Input: part model. Units: mm. Frame: model coordinates. Give positions to 0.01 mm unless a question says otherwise; leave off trailing zeros. Write each loop counter-clockwise with the first axis right and the second up, starting at its lowest first coordinate (ties: lowest second). Pieces come first, ordered by that corner, then holes. Notation, with made-up numbers: (8, 9) -> (27, 9) arc R29 ccw to (27, 39) -> close; hole circle Ø1 at (61, 45.5). An arc over 180 degrees is marked (long way). Return JSON: item names as keys, results as strings. Group by question number.
Item 1: Section B-B, the plane z = 2. Return loops of the section in (x, y).
Item 2: Section C-C, the plane y = 12.5. Return loops of the section in (x, z) (3 decimals).
Item 3: Line query: line 1 (X direction, y = 34, z = 5.5); line 2 (X direction, y = 21, z = 4.75); line 3 (Y direction, x = 29.5, z = 5.5). Output: solid intervals per line, ascending. Write a range as [from, to].
Item 4: Pin query (flat end, axial travel): P1, Ø3, axis at x = 35, z = 4.5, coming from the -Y side; P2, Ø1, axis at x = 8.5, z = 3, coming from the +Y side. Return the tip coordinate at first contact, or that it passes through.
Item 5: Section A-A, the plane x = 34. Return loops of the section in (y, z) (3 decimals).
Item 6: Section D-D, the plane y = 0. Return loops of the section in (x, z) (3 decimals), then the cut area to 3 significant figures.
from build123d import *

# Parameters (mm, degrees)
F0_R     = 50.8
F1_DEPTH = 6.35
F3_DEPTH = 3.175


with BuildPart() as f1:
    # F0 (on Top) → F1 (new body)
    with BuildSketch(Plane.XY):
        Circle(F0_R)
    extrude(amount=F1_DEPTH)

    # F2 (on face) → F3 (cut)
    with BuildSketch(Plane.XY.offset(6.35)):
        with BuildLine():
            ThreePointArc((15.112324, 8.831488), (3.651467, 2.698075), (-9.320416, 3.53488))
            ThreePointArc((-9.320416, 3.53488), (-32.253054, -21.213472), (-4.365525, -40.204853))
            ThreePointArc((-4.365525, -40.204853), (9.25251, -39.514444), (22.098763, -34.942649))
            ThreePointArc((22.098763, -34.942649), (17.400158, -35.046174), (12.701553, -34.942649))
            ThreePointArc((12.701553, -34.942649), (9.453009, -34.523417), (7.319516, -32.038059))
            ThreePointArc((7.319516, -32.038059), (15.827852, -28.814343), (24.832496, -27.510311))
            ThreePointArc((24.832496, -27.510311), (32.746976, -25.459085), (38.501162, -19.650828))
            ThreePointArc((38.501162, -19.650828), (40.771781, -15.886564), (41.832902, -11.620486))
            ThreePointArc((41.832902, -11.620486), (33.877001, -16.787957), (24.832496, -19.650828))
            ThreePointArc((24.832496, -19.650828), (29.815505, -13.430648), (35.254855, -7.605316))
            ThreePointArc((35.254855, -7.605316), (41.278783, 12.303986), (31.977173, 30.909041))
            ThreePointArc((31.977173, 30.909041), (35.554887, 23.205066), (35.254855, 14.716176))
            ThreePointArc((35.254855, 14.716176), (15.477583, 39.467908), (-16.163122, 41.097168))
            ThreePointArc((-16.163122, 41.097168), (-7.968292, 40.127246), (0, 37.98195))
            ThreePointArc((0, 37.98195), (2.887171, 36.599375), (4.963089, 34.162607))
            ThreePointArc((4.963089, 34.162607), (-1.010732, 31.624663), (-7.500219, 31.505231))
            ThreePointArc((-7.500219, 31.505231), (-1.491468, 29.04792), (4.963089, 29.742295))
            ThreePointArc((4.963089, 29.742295), (7.619099, 31.6133), (10.671567, 32.725722))
            ThreePointArc((10.671567, 32.725722), (14.857029, 32.055581), (17.791109, 28.99644))
            ThreePointArc((17.791109, 28.99644), (19.347167, 23.888888), (18.469164, 18.622248))
            ThreePointArc((18.469164, 18.622248), (15.14181, 21.198982), (12.786984, 24.68691))
            ThreePointArc((12.786984, 24.68691), (17.163098, 13.855457), (27.56623, 8.540798))
            ThreePointArc((27.56623, 8.540798), (26.557747, 5.699635), (26.028505, 2.731615))
            ThreePointArc((26.028505, 2.731615), (24.468311, -0.799827), (21.415329, -3.162999))
            ThreePointArc((21.415329, -3.162999), (20.44222, 2.261754), (21.415329, 7.686506))
            ThreePointArc((21.415329, 7.686506), (19.491688, 5.874092), (18.169021, 3.585906))
            ThreePointArc((18.169021, 3.585906), (16.975731, -0.906667), (16.973011, -5.555016))
            ThreePointArc((16.973011, -5.555016), (16.032075, -11.360599), (12.616124, -16.148232))
            ThreePointArc((12.616124, -16.148232), (6.875784, -18.260537), (2.127092, -14.405247))
            ThreePointArc((2.127092, -14.405247), (3.95514, -10.785374), (7.252841, -8.425204))
            ThreePointArc((7.252841, -8.425204), (13.847913, -1.010771), (15.112324, 8.831488))
        make_face()
        with BuildLine():
            ThreePointArc((-23.696838, 23.682131), (-19.798362, 29.346782), (-13.441595, 31.969357))
            ThreePointArc((-13.441595, 31.969357), (-16.672015, 37.73461), (-23.107406, 36.231447))
            ThreePointArc((-23.107406, 36.231447), (-29.15748, 31.539036), (-32.012127, 24.434594))
            ThreePointArc((-32.012127, 24.434594), (-28.736741, 26.680977), (-25.31456, 28.696684))
            ThreePointArc((-25.31456, 28.696684), (-24.969334, 27.114262), (-24.609111, 25.535187))
            ThreePointArc((-24.609111, 25.535187), (-24.317241, 24.527789), (-23.696838, 23.682131))
        make_face()
        with BuildLine():
            ThreePointArc((-9.197756, 25.535187), (-6.724581, 24.427669), (-5.085402, 22.269826))
            ThreePointArc((-5.085402, 22.269826), (-3.220597, 19.405613), (-0.489241, 17.351128))
            ThreePointArc((-0.489241, 17.351128), (2.029713, 17.241099), (4.510092, 17.693825))
            ThreePointArc((4.510092, 17.693825), (6.713953, 19.342602), (8.158797, 21.685228))
            ThreePointArc((8.158797, 21.685228), (8.296615, 23.240133), (7.715309, 24.688859))
            ThreePointArc((7.715309, 24.688859), (5.068899, 26.392475), (2.212011, 25.071872))
            ThreePointArc((2.212011, 25.071872), (1.166697, 24.006752), (0, 23.076171))
            ThreePointArc((0, 23.076171), (-1.454137, 22.680928), (-2.908273, 23.076171))
            ThreePointArc((-2.908273, 23.076171), (-4.628321, 24.658533), (-6.657773, 25.817741))
            ThreePointArc((-6.657773, 25.817741), (-7.961822, 25.982624), (-9.197756, 25.535187))
        make_face()
    extrude(amount=-F3_DEPTH, mode=Mode.SUBTRACT)


solid = f1.part
Answer below:
{
 "1": {"outline": "circle Ø101.6 at (0, 0)"},
 "2": {"outline": "(-49.238, 0) -> (49.238, 0) -> (49.238, 6.35) -> (41.261, 6.35) -> (41.261, 3.175) -> (18.557, 3.175) -> (18.557, 6.35) -> (-49.238, 6.35) -> close"},
 "3": {"line 1": "x = [-37.74, -26.8], [-13.55, 4.72], [23.47, 37.74]", "line 2": "x = [-46.26, -4.43], [7.86, 13.3], [15.33, 19.18], [33.05, 35.86], [39.11, 46.26]", "line 3": "y = [-41.36, -26.86], [-18.51, -13.8], [27.24, 41.36]"},
 "4": {"P1": "stops at y = -38.19", "P2": "stops at y = 50.17"},
 "5": {"outline": "(-37.744, 0) -> (37.744, 0) -> (37.744, 6.35) -> (28.912, 6.35) -> (28.912, 3.175) -> (27.727, 3.175) -> (27.727, 6.35) -> (18.694, 6.35) -> (18.694, 3.175) -> (-8.872, 3.175) -> (-8.872, 6.35) -> (-16.73, 6.35) -> (-16.73, 3.175) -> (-24.656, 3.175) -> (-24.656, 6.35) -> (-37.744, 6.35) -> close"},
 "6": {"outline": "(-50.8, 0) -> (50.8, 0) -> (50.8, 6.35) -> (39.573, 6.35) -> (39.573, 3.175) -> (25.018, 3.175) -> (25.018, 6.35) -> (20.607, 6.35) -> (20.607, 3.175) -> (17.118, 3.175) -> (17.118, 6.35) -> (14.269, 6.35) -> (14.269, 3.175) -> (-22.196, 3.175) -> (-22.196, 6.35) -> (-50.8, 6.35) -> close", "area": "472 mm2"}
}
